Check sheet for the modelled part. Datum: model origin and axes. Units: mm. A direction names the side the tool comes from. Round coordinates to 2 decimals unless told otherwise and drop trailing zeros. Answer as a JSON object with one key per item and string values. Group by question number.
Item 1: Release check for a two-part mould opening along X. For faces 3 (the cylindrical face through (79.4, 3.01, -55.43)), 4 (the cylindrical face through (66.583, 4.028, -10.759)), 5 (the cylindrical face through (0.57, 3.01, -0.6)) record: pulls with the +X half, pulls with the -X half, needs draft (parallel to the pull), parting line crosses it, or undercut.
Item 2: Set-up check for faces 1 (the cylindrical face through (48.365, 4.028, -48.58)), 2 (the cylindrical face through (72.727, 1.014, -10.358)): record each of +Z, -Z, +X, -X, +Y, -Y from which the full face is reachable in a straight line by a thin tool's end or side.
Item 3: Gauge pin test, flat ends, axial feed: P1, Ø7.5, axis at x = 56.5, z = -47, coming from the +Y side; P2, Ø4, axis at x = 70, z = -46, coming from the -Y side. Record the tip position at first contact, or that the pin passes through.
Item 4: Sectioned sample at A-A on z = -46. Count the separate pieces of the cut face and the enclosed holes in it, plus the area to 3 significant figures.
Item 5: Thickness scan on line 1 (Z direction, x = 24, y = 1.4); line 2 (Y direction, x = 23, z = -13); line 3 (Z direction, x = 8.5, y = 4.25). Record the ranges inside material, lowest first.
```python
from build123d import *

# Parameters (mm, degrees)
SKETCH2_W            = 80
SKETCH2_H            = 56
BOSS_EXTRUDE1_DEPTH  = 6
SKETCH3_R            = 3.5
CUT_EXTRUDE1_DEPTH   = 4
SKETCH4_R            = 2.75
CUT_EXTRUDE2_DEPTH   = 98.836598469
LPATTERN1_COUNT      = 6
LPATTERN1_PITCH      = 12
LPATTERN1_COUNT_DIR2 = 4
LPATTERN1_PITCH_DIR2 = 12
FILLET1_R            = 2


with BuildPart() as part:
    # Sketch2 → Boss-Extrude1 (new body)
    with BuildSketch(Plane(origin=(0, 0, 0), x_dir=(1, 0, 0), z_dir=(0, 1, 0))):
        with Locations((40, 28)):
            Rectangle(SKETCH2_W, SKETCH2_H)
    extrude(amount=BOSS_EXTRUDE1_DEPTH)

    # Sketch3 → Cut-Extrude1 (cut)
    with BuildSketch(Plane(origin=(0, 6, 0), x_dir=(1, 0, 0), z_dir=(0, 1, 0))):
        with Locations(Location((10, 46, 0), (0, 0, 270))):
            Circle(SKETCH3_R)
    cut_extrude1 = extrude(amount=-CUT_EXTRUDE1_DEPTH, mode=Mode.SUBTRACT)

    # Sketch4 → Cut-Extrude2 (cut, through all)
    with BuildSketch(Plane(origin=(0, 6, 0), x_dir=(1, 0, 0), z_dir=(0, 1, 0))):
        with Locations(Location((10, 46, 0), (0, 0, 270))):
            Circle(SKETCH4_R)
    cut_extrude2 = extrude(amount=-CUT_EXTRUDE2_DEPTH, mode=Mode.SUBTRACT)

    # LPattern1: Cut-Extrude1, Cut-Extrude2 6 × 4
    with Locations(*[(i * LPATTERN1_PITCH, 0, j * LPATTERN1_PITCH_DIR2) for i in range(LPATTERN1_COUNT) for j in range(LPATTERN1_COUNT_DIR2) if (i, j) != (0, 0)]):
        add(cut_extrude1, mode=Mode.SUBTRACT)
        add(cut_extrude2, mode=Mode.SUBTRACT)

    # Fillet1
    fillet1_edges = [part.edges().sort_by_distance(p)[0] for p in [
        (80, 6, -28),
        (40, 6, -56),
        (0, 6, -28),
        (40, 0, -56),
        (80, 0, -28),
        (40, 0, 0),
        (0, 0, -28),
        (0, 3, -56),
        (80, 3, -56),
        (80, 3, 0),
        (0, 3, 0),
        (40, 6, 0),
    ]]
    fillet(fillet1_edges, radius=FILLET1_R)


solid = part.part
```
Completed:
{
 "1": {"face 3": "pulls with the +X half", "face 4": "undercut", "face 5": "pulls with the -X half"},
 "2": {"face 1": "+Y", "face 2": "+Y, -Y"},
 "3": {"P1": "y = 6", "P2": "through"},
 "4": {"separate pieces": "7", "enclosed holes": "0", "area": "243 mm²"},
 "5": {"line 1": "-55.91 to -47.89, -44.11 to -35.89, -32.11 to -23.89, -20.11 to -11.89, -8.11 to -0.09", "line 2": "0 to 2", "line 3": "-55.98 to -49.16, -42.84 to -37.16, -30.84 to -25.16, -18.84 to -13.16, -6.84 to -0.02"}
}
